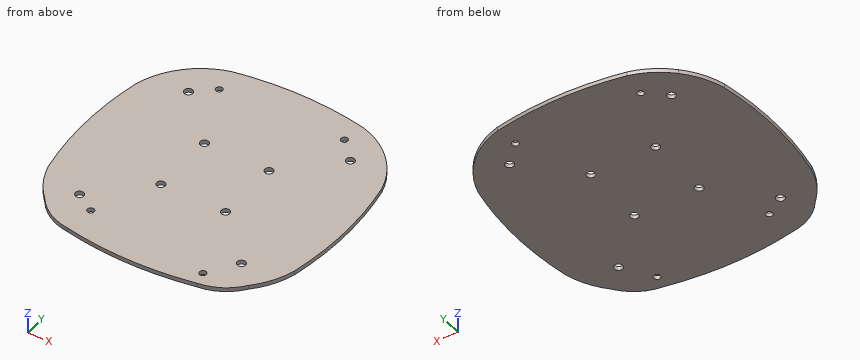
Autodesk Inventor part; units mm, degrees
ref_plane "YZ Plane" through (0, 0, 0) normal (1, 0, 0) x (0, 1, 0)
ref_plane "XZ Plane" through (0, 0, 0) normal (0, 1, 0) x (-1, 0, 0)
ref_plane "XY Plane" through (0, 0, 0) normal (0, 0, 1) x (1, 0, 0)
sketch "Sketch1" plane through (0, 0, 0) normal (0, 0, 1) x (1, 0, 0)
  line L0 (0, 3.1673) -> (0, -2.4908)
  spline S0 degree 2 poles (-48.26, -25.4) (-53.34, 0) (-48.26, 25.4) knots 0 0 0 1 1 1
  line L1 (-20.5368, 0) -> (25.7294, 0)
  line L2 (0, 0) -> (-9.8402, -9.8402)
  line L3 (0, 0) -> (13.9161, 0) construction
  line L4 (0, 0) -> (-23.2805, 23.2805)
  arc A0 (-39.9068, 39.9068) -> (-48.26, 25.4) centre (-17.1376, 17.1376) ccw
  arc A1 (-48.26, -25.4) -> (-39.9068, -39.9068) centre (-17.1376, -17.1376) ccw
  spline S1 degree 2 poles (48.26, -25.4) (53.34, 0) (48.26, 25.4) knots 0 0 0 1 1 1
  arc A2 (48.26, 25.4) -> (39.9068, 39.9068) centre (17.1376, 17.1376) ccw
  arc A3 (39.9068, -39.9068) -> (48.26, -25.4) centre (17.1376, -17.1376) ccw
  spline S2 degree 2 poles (25.476, -48.26) (-0.0768, -53.34) (-25.476, -48.26) knots 0 0 0 1 1 1
  arc A4 (-39.9068, -39.9068) -> (-25.476, -48.26) centre (-23.264, -27.7968) ccw
  arc A5 (25.476, -48.26) -> (39.9068, -39.9068) centre (23.264, -27.7968) ccw
  spline S3 degree 2 poles (-25.4, 48.26) (0, 53.34) (25.4, 48.26) knots 0 0 0 1 1 1
  arc A6 (39.9068, 39.9068) -> (25.4, 48.26) centre (17.1376, 17.1376) ccw
  arc A7 (-25.4, 48.26) -> (-39.9068, 39.9068) centre (-17.1376, 17.1376) ccw
  point P0 (-50.8, 0)
  point P1 (50.8, 0)
  point P2 (-0.076, -50.8)
  point P3 (0, 50.8)
  point P4 (-12.7, 12.7)
  point P5 (-31.75, 31.75)
  point P6 (-31.75, -31.75)
  point P7 (-12.7, -12.7)
  point P8 (12.7, 12.7)
  point P9 (31.75, 31.75)
  point P10 (31.75, -31.75)
  point P11 (12.7, -12.7)
  point P12 (24.13, -42.935)
  point P13 (24.13, 39.615)
  point P14 (-24.13, 38.345)
  point P15 (-24.13, -36.585)
  dimension "d23" = 1.5875
  dimension "d24" = 0
  dimension "d1" = 45
  dimension "d6" = 50.8
  dimension "d7" = 25.4
  dimension "d8" = 48.26
  dimension "d15" = 48.26
  dimension "d16" = 50.8
  dimension "d17" = 25.4
  dimension "d19" = 25.4
  dimension "d20" = 50.8
  dimension "d21" = 48.26
  dimension "d22" = 25.4
  dimension "d25" = 12.7
  dimension "d26" = 31.75
  dimension "d34" = 48.26
  dimension "d38" = 48.26
  dimension "d39" = 6.35
  dimension "d40" = 82.55
  dimension "d41" = 1.27
  dimension "d42" = 48.26
  dimension "d43" = 0
  dimension "d44" = 24.13
extrude "Extrusion1" add sketch "Sketch1" along normal blind 1.5875
hole "Hole1" at (-12.7, 12.7, 0) at (-31.75, 31.75, 0) at (-31.75, -31.75, 0) at (-12.7, -12.7, 0) at (31.75, 31.75, 0) at (12.7, 12.7, 0) at (12.7, -12.7, 0) at (31.75, -31.75, 0) direction (0, 0, 1) diameter 3.302 end through all
hole "Hole2" at (24.13, -42.935, 0) at (24.13, 39.615, 0) at (-24.13, 38.345, 0) at (-24.13, -36.585, 0) direction (0, 0, 1) diameter 2.6416 end through all
equation "\"d15\" = d8"
equation "\"d21\" = d8"
properties part number "Base"
Geometry: final body of the model. Coordinates: model frame, mm. Give positions to 0.01 mm unless a question says otherwise; leave off trailing zeros. Write each loop counter-clockwise with the first axis right and the second up, starting at its lowest first coordinate (ties: lowest second). Pieces come first, ordered by that corner, then holes.
(1) Cut plane B-B, the plane x = -31.75. Return loops of the section in (y, z), then the cut area to 3 significant figures.
(2) Cut plane A-A, the plane y = 31.75. Return loops of the section in (x, z).
(3) Ray query, line 1 (X direction, y = -31.75, z = 0.3); line 2 (X direction, y = -12.7, z = 1.2) (3 decimals); line 3 (Y direction, x = -14, z = 0.7). Return the intervals inside material, ascending.
(4) First-contact query: P1, Ø2.5, axis at x = 24.13, y = -42.935, coming from the +Z side. Flat tip, straight axial feed; report the tip coordinate or a pass-through.
(5) Cut plane C-C, the plane z = 1. Give the number of separate pieces and of enclosed holes in the cut face, then the cut area to 3 significant figures.
Values follow:
1. outline: (-46.55, 0) - (-33.4, 0) - (-33.4, 1.59) - (-46.55, 1.59) - close; (-30.1, 0) - (30.1, 0) - (30.1, 1.59) - (-30.1, 1.59) - close; (33.4, 0) - (45.83, 0) - (45.83, 1.59) - (33.4, 1.59) - close
1. area: 136 mm2
2. outline: (-45.83, 0) - (-33.4, 0) - (-33.4, 1.59) - (-45.83, 1.59) - close; (-30.1, 0) - (30.1, 0) - (30.1, 1.59) - (-30.1, 1.59) - close; (33.4, 0) - (45.83, 0) - (45.83, 1.59) - (33.4, 1.59) - close
3. line 1: x = -45.83 to -33.4, -30.1 to 30.1, 33.4 to 45.83
3. line 2: x = -50.165 to -14.351, -11.049 to 11.049, 14.351 to 50.165
3. line 3: y = -50.04 to -13.72, -11.68 to 11.68, 13.72 to 50.03
4. P1: passes through
5. separate pieces: 1
5. enclosed holes: 12
5. area: 8,920 mm2
